from build123d import *

# Parameters (mm, degrees)
F0_W     = 50
F0_H     = 40
F1_DEPTH = 20
F2_W     = 48
F2_H     = 38
F3_DEPTH = 19
F4_W     = 5
F4_H     = 5
F5_DEPTH = 19
F6_R     = 1.5
F7_DEPTH = 10


with BuildPart() as f1:
    # F0 (on Top) → F1 (new body)
    with BuildSketch(Plane.XY):
        with Locations((-36.687503, 37.0625)):
            Rectangle(F0_W, F0_H)
    extrude(amount=F1_DEPTH)

    # F2 (on face) → F3 (cut)
    with BuildSketch(Plane.XY.offset(20)):
        with Locations((-36.687503, 37.0625)):
            Rectangle(F2_W, F2_H)
    extrude(amount=-F3_DEPTH, mode=Mode.SUBTRACT)

    # F4 (on face) → F5 (join)
    with BuildSketch(Plane.XY.offset(1)):
        with Locations((-15.187503, 53.5625)):
            Rectangle(F4_W, F4_H)
        with Locations((-15.187503, 20.5625)):
            Rectangle(F4_W, F4_H)
        with Locations((-58.187503, 20.5625)):
            Rectangle(F4_W, F4_H)
        with Locations((-58.187503, 53.5625)):
            Rectangle(F4_W, F4_H)
    extrude(amount=F5_DEPTH)

    # F6 (on face) → F7 (cut)
    with BuildSketch(Plane.XY.offset(20)):
        with Locations((-15.187503, 53.5625)):
            Circle(F6_R)
        with Locations((-15.187503, 20.5625)):
            Circle(F6_R)
        with Locations((-58.187503, 20.5625)):
            Circle(F6_R)
        with Locations((-58.187503, 53.5625)):
            Circle(F6_R)
    extrude(amount=-F7_DEPTH, mode=Mode.SUBTRACT)


solid = f1.part
Build history of the part. All positions in model axes, mm. A direction names the side the tool comes from. Give positions to 0.01 mm unless a question says otherwise; leave off trailing zeros. Loops run counter-clockwise (first coordinate to the right, second up) from the corner with the lowest first, then second, coordinate; pieces in that order, holes last. Notation, with made-up numbers: (76.25, -32.5) - (86.25, -32.5) arc R7 ccw to (86.25, -27.5) - close; hole circle Ø9 at (89, -32). An arc over 180 degrees is marked (long way). Write item = value, one per line. Start each with the question number.
1) Probe probe 1 along X at (y, z) = (30, 3.75); probe 2 along Y at (x, z) = (-15, 16.25); probe 3 along Y at (x, z) = (-26.5, 4.25). List the from-to ranges inside material, lowest first. Write a range as from..to.
2) Tool access for faces 1 (the flat face through (-37, 37, 0)), 2 (the cylindrical face through (-56.8, 52.99, 15.07)): list every direction of +Z, -Z, +X, -X, +Y, -Y with a clear straight run to the whole face (end or side of a thin tool).
3) Drop flat-ended pins along their axis: pin 1 Ø8 at (x, y) = (-33, 32.5) entering from +Z; pin 2 Ø4 at (x, y) = (-15.19, 53.56) entering from +Z; pin 3 Ø2.5 at (x, y) = (-58, 20.5) entering from +Z. Give the stop position or say it passes through.
4) Band-saw the part on C-C on x = -24.5. Give the cut face in (y, z).
5) Band-saw the part on D-D on z = 18.5. Give the cut face in (x, y), plus the area to 3 significant figures.
6) Band-saw the part on B-B on z = 7.5. Give the cut face in (x, y), plus the area to 3 significant figures.
7) Band-saw the part on A-A on y = 42. Give the cut face in (x, z), plus the area to 3 significant figures.
8) Pull direction X, two halves, no side cores. Call faces 3 (the flat face through (-37, 17.062, 10)), 4 (the flat face through (-37, 56.062, 11)), 5 (the flat face through (-11.688, 37, 10)), 6 (the cylindrical face through (-14.381, 21.827, 15.07)): +X half, -X half, draft (parallel to the pull), parting line (faces both ways), or undercut.
Final values:
q1.probe_1 = -61.69..-60.69, -12.69..-11.69
q1.probe_2 = 17.06..19.07, 22.05..23.06, 51.06..52.07, 55.05..57.06
q1.probe_3 = 17.06..18.06, 56.06..57.06
q2.face_1 = -Z, +X, -X, +Y, -Y
q2.face_2 = +Z
q3.pin_1 = 1
q3.pin_2 = 20
q3.pin_3 = 10
q4.outline = (17.06, 0) - (57.06, 0) - (57.06, 20) - (56.06, 20) - (56.06, 1) - (18.06, 1) - (18.06, 20) - (17.06, 20) - close
q5.outline = (-61.69, 17.06) - (-11.69, 17.06) - (-11.69, 57.06) - (-61.69, 57.06) - close; hole (-60.69, 23.06) - (-55.69, 23.06) - (-55.69, 18.06) - (-17.69, 18.06) - (-17.69, 23.06) - (-12.69, 23.06) - (-12.69, 51.06) - (-17.69, 51.06) - (-17.69, 56.06) - (-55.69, 56.06) - (-55.69, 51.06) - (-60.69, 51.06) - close; hole circle Ø3 at (-58.19, 20.56); hole circle Ø3 at (-58.19, 53.56); hole circle Ø3 at (-15.19, 20.56); hole circle Ø3 at (-15.19, 53.56)
q5.area = 248 mm²
q6.outline = (-61.69, 17.06) - (-11.69, 17.06) - (-11.69, 57.06) - (-61.69, 57.06) - close; hole (-60.69, 23.06) - (-55.69, 23.06) - (-55.69, 18.06) - (-17.69, 18.06) - (-17.69, 23.06) - (-12.69, 23.06) - (-12.69, 51.06) - (-17.69, 51.06) - (-17.69, 56.06) - (-55.69, 56.06) - (-55.69, 51.06) - (-60.69, 51.06) - close
q6.area = 276 mm²
q7.outline = (-61.69, 0) - (-11.69, 0) - (-11.69, 20) - (-12.69, 20) - (-12.69, 1) - (-60.69, 1) - (-60.69, 20) - (-61.69, 20) - close
q7.area = 88.0 mm²
q8.face_3 = draft
q8.face_4 = undercut
q8.face_5 = +X half
q8.face_6 = undercut
